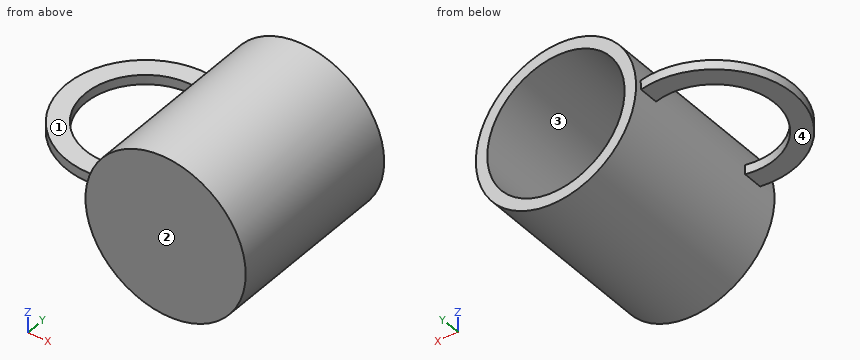
from build123d import *

# Parameters (mm, degrees)
CROQUIS1_R              = 42
CROQUIS1_R_2            = 36
SALIENTE_EXTRUIR1_DEPTH = 95
CROQUIS2_R              = 42
SALIENTE_EXTRUIR2_DEPTH = 5
EXTRUIR_L_MINA1_DEPTH   = 5


with BuildPart() as part:
    # Croquis1 → Saliente-Extruir1 (new body)
    with BuildSketch(Plane(origin=(0, 0, 0), x_dir=(1, 0, 0), z_dir=(0, 1, 0))):
        Circle(CROQUIS1_R)
        Circle(CROQUIS1_R_2, mode=Mode.SUBTRACT)
    extrude(amount=SALIENTE_EXTRUIR1_DEPTH)

    # Croquis2 → Saliente-Extruir2 (add)
    with BuildSketch(Plane.XZ):
        Circle(CROQUIS2_R)
    extrude(amount=-SALIENTE_EXTRUIR2_DEPTH)

    # Croquis3 → Extruir-Lámina1 (add)
    with BuildSketch(Plane.XY):
        with BuildLine():
            ThreePointArc((-42, 81.333269167), (-80.835192592, 50.726606051), (-42, 20.119942936))
            Line((-42, 20.119942936), (-39.662910525, 10.396876918))
            ThreePointArc((-39.662910525, 10.396876918), (-90.835192592, 50.726606051), (-39.662910525, 91.056335185))
            Line((-39.662910525, 91.056335185), (-42, 81.333269167))
        make_face()
    extrude(amount=EXTRUIR_L_MINA1_DEPTH)


solid = part.part
Design review of the part built by this model. Coordinates are the model's own, in mm. Face numbers are marked on the shaded views. A direction names the side the tool comes from. Coordinates: 2 decimals unless noted, no trailing zeros. Write each loop counter-clockwise with the first axis right and the second up, starting at its lowest first coordinate (ties: lowest second). Pieces come first, ordered by that corner, then holes. Notation, with made-up numbers: (71, -4.75) -> (107, -4.75) arc R15 cw to (107, 15.25) -> close; hole circle Ø6 at (-17, 21). An arc over 180 degrees is marked (long way). Write each question's results on one line, items separated by ' | '. Start each with the question number.
(1) Tool access review of the marked faces 1 and 2: name each direction out of +Z, -Z, +X, -X, +Y, -Y from which nothing blocks a thin tool from reaching the whole face with its end or side.
(2) The part is to be moulded in two halves that separate along X. For the marked faces 3 and 4, say which applies: pulls with the +X half, pulls with the -X half, needs draft (parallel to the pull), parting line crosses it, or undercut.
(3) Take a section at A-A on x = -64. Write out the cut boundary in (y, z), and give its area (3 significant figures).
(4) For line 1 along Y through (x, z) = (-30.5, -15); line 2 along X through (y, z) = (23.5, 19.5); line 3 along X through (y, z) = (43, -16), list the stretches that pass through material, from the lowest coordinate up. Write a range as from..to.
(5) Take a section at C-C on x = 0. Write out the cut boundary in (y, z).
(6) Clearance check with flat-ended pins moving along their axes: P1, Ø1, axis at y = 40, z = -33.5, coming from the +X side; P2, Ø8, axis at y = 48, z = -9, coming from the +X side; P3, Ø2, axis at y = 18, z = 2, coming from the +X side. State where each tip first meets the part, or that it passes through.
(7) Take a section at B-B on y = 79. Write out the cut boundary in (x, z), and give its area (3 significant figures).
(8) Take a section at D-D on y = 68. Write out the cut boundary in (x, z), and give its area (3 significant figures).
Results found:
1) face 1: +Z, -X, +Y, -Y | face 2: +Z, -Z, +X, -X, -Y
2) face 3: undercut | face 4: needs draft
3) outline: (11.92, 0) -> (22.86, 0) -> (22.86, 5) -> (11.92, 5) -> close; (78.59, 0) -> (89.53, 0) -> (89.53, 5) -> (78.59, 5) -> close | area: 109 mm2
4) line 1: y = 0..5 | line 2: x = -37.2..-30.26, 30.26..37.2 | line 3: x = -38.83..-32.25, 32.25..38.83
5) outline: (0, -42) -> (95, -42) -> (95, -36) -> (5, -36) -> (5, 36) -> (95, 36) -> (95, 42) -> (0, 42) -> close
6) P1: stops at x = 25.98 | P2: stops at x = 41.7 | P3: stops at x = 41.99
7) outline: (-79.71, 0) -> (-63.2, 0) -> (-63.2, 5) -> (-79.71, 5) -> close; circle Ø84 at (0, 0); hole circle Ø72 at (0, 0) | area: 1,550 mm2
8) outline: (-87.07, 0) -> (-75.67, 0) -> (-75.67, 5) -> (-87.07, 5) -> close; circle Ø84 at (0, 0); hole circle Ø72 at (0, 0) | area: 1,530 mm2
